Source: three-view drawing plus pictorial views. Frame: mm from the lowest corner of the part. Give positions to 0.01 mm unless a question says otherwise; leave off trailing zeros. Loops run counter-clockwise (first coordinate to the right, second up) from the corner with the lowest first, then second, coordinate; pieces in that order, holes last. Notation, with made-up numbers: (26, -5) - (49, -5) arc R30 cw to (49, 25) - close; hole circle Ø1 at (-29, -19). An arc over 180 degrees is marked (long way). Answer in a Markdown table with one row per item.
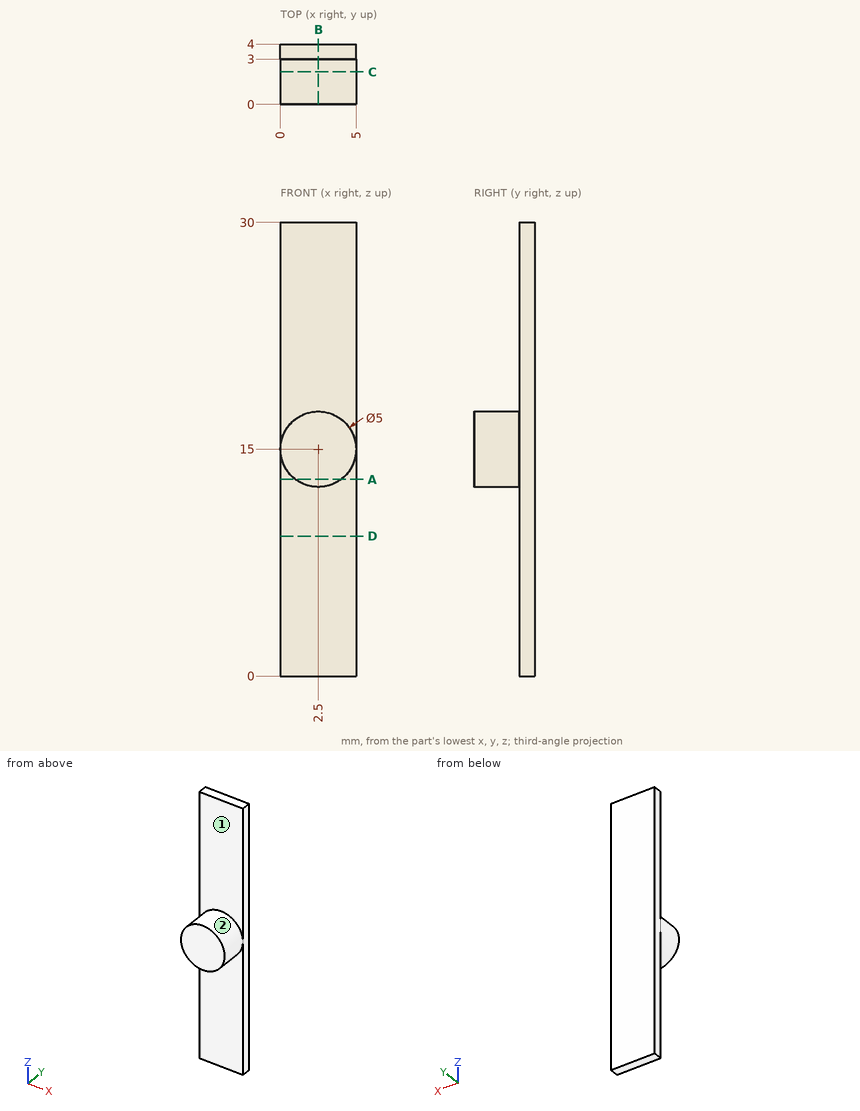
Q1. Cut plane D-D (z = 9.25). Output: boundary loops of the cut face in (x, y).
Check values:
| item | result |
|---|---|
| outline | (0, 3) - (5, 3) - (5, 4) - (0, 4) - close |
Q2. Cut plane A-A (z = 13). Output: boundary loops of the cut face in (x, y).
Check values:
| item | result |
|---|---|
| outline | (0, 3) - (1, 3) - (1, 0) - (4, 0) - (4, 3) - (5, 3) - (5, 4) - (0, 4) - close |
Q3. Material intervals for line 1 along Y through (x, z) = (3, 23.5); line 2 along Z through (x, y) = (3.25, 1.35); line 3 along Z through (x, y) = (3.45, 2.25), sorted ascending.
Check values:
| item | result |
|---|---|
| line 1 | 3 to 4 |
| line 2 | 12.62 to 17.38 |
| line 3 | 12.69 to 17.31 |
Q4. Draft query along X for the marked faces 1 and 2. Return one class per face: pulls with the +X half, pulls with the -X half, needs draft (parallel to the pull), parting line crosses it, or undercut.
Check values:
| item | result |
|---|---|
| face 1 | needs draft |
| face 2 | parting line crosses it |
Q5. First-contact query: pin 1 (1 mm diameter, centred on x = 3, y = 1, fed in from -Z); pin 2 (2.5 mm diameter, centred on x = 2, z = 26, fed in from -Y). Flat tips, straight axial feed; report the tip coordinate or a pass-through.
Check values:
| item | result |
|---|---|
| pin 1 | z = 12.5 |
| pin 2 | y = 3 |
Q6. Cut plane C-C (y = 2.15). Output: boundary loops of the cut face in (x, z), and give its area (3 significant figures).
Check values:
| item | result |
|---|---|
| outline | circle Ø5 at (2.5, 15) |
| area | 19.6 mm² |
Q7. Cut plane B-B (x = 2.5). Output: boundary loops of the cut face in (y, z).
Check values:
| item | result |
|---|---|
| outline | (0, 12.5) - (3, 12.5) - (3, 0) - (4, 0) - (4, 30) - (3, 30) - (3, 17.5) - (0, 17.5) - close |
